Geometry check sheet. Reference: the model listing, model coordinates, mm. Face numbers are marked on the shaded views. A direction names the side the tool comes from. Round coordinates to 2 decimals unless told otherwise and drop trailing zeros. Write each loop counter-clockwise with the first axis right and the second up, starting at its lowest first coordinate (ties: lowest second). Pieces come first, ordered by that corner, then holes. Notation, with made-up numbers: M 42.5,18 L 63.5,18 A26 ccw 63.5,42 Z; hole C -35.5,4 d10. An arc over 180 degrees is marked long. One line per item, written item: value. Start each with the question number.
1. Scan lines: probe 1 along X at (y, z) = (20.5, 17); probe 2 along Z at (x, y) = (8, 2); probe 3 along Y at (x, z) = (33, -2). Record each from-to range of solid material in increasing order. Write a range as [from, to].
2. Depth check by flat-ended pin: P1, Ø12.5, axis at x = 16.5, z = -32, coming from the +Y side; P2, Ø1.1, axis at x = 42.5, z = -40, coming from the -Y side. Enter the tip coordinate at first touch or a pass-through.
3. Access from +Z, -Z, +X, -X, +Y, -Y to the whole of each face (thin tool, end or side, straight path). Record for the marked faces 1 and 2.
4. Section check A-A (x = -21.8). Record the boundary of the cut face in (y, z), and give its area (3 significant figures).
5. Section check C-C (y = 14.5). Count the separate pieces of the cut face and the enclosed holes in it, and give its area (3 significant figures).
6. Section check B-B (z = -6.5). Record the boundary of the cut face in (x, y), and give its area (3 significant figures).
7. Section check D-D (x = 33). Record the boundary of the cut face in (y, z).
8. Release check for a two-part mould opening along X. For the marked faces 3, 4, 5 and 6 record: pulls with the +X half, pulls with the -X half, needs draft (parallel to the pull), parting line crosses it, or undercut.
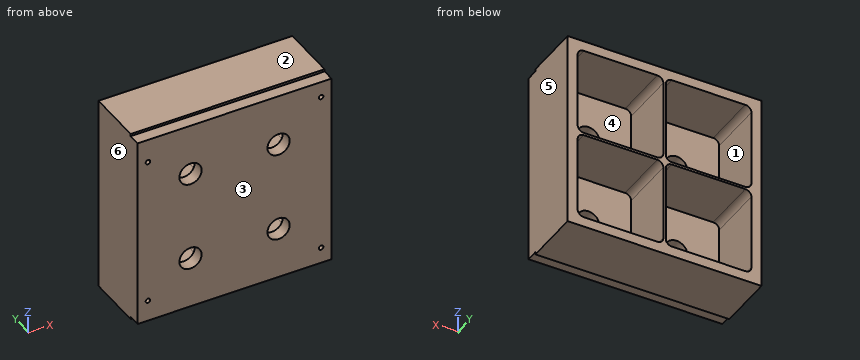
from build123d import *

# Parameters (mm, degrees)
SKETCH1_W           = 96
SKETCH1_H           = 98.4
BOSS_EXTRUDE1_DEPTH = 28
FILLET1_R           = 3
SKETCH2_W           = 96
SKETCH2_H           = 96
BOSS_EXTRUDE2_DEPTH = 6
SKETCH4_R           = 1.1305
CUT_EXTRUDE2_DEPTH  = 4.7
SKETCH6_R           = 5.5
CUT_EXTRUDE3_DEPTH  = 75.22021288


with BuildPart() as part:
    # Sketch1 → Boss-Extrude1 (new body)
    with BuildSketch(Plane(origin=(0, 0, 0), x_dir=(1, 0, 0), z_dir=(0, 1, 0))):
        Rectangle(SKETCH1_W, SKETCH1_H)
        Polygon((-43, -44.2), (-43, -0.6), (-0.6, -0.615), (-0.6, -44.2), align=None, mode=Mode.SUBTRACT)
        Polygon((-43, 44.2), (-0.6, 44.2), (-0.6, 0.615), (-43, 0.6), align=None, mode=Mode.SUBTRACT)
        Polygon((43, -44.2), (43, -0.6), (0.6, -0.615), (0.6, -44.2), align=None, mode=Mode.SUBTRACT)
        Polygon((0.6, 44.2), (43, 44.2), (43, 0.6), (0.6, 0.615), align=None, mode=Mode.SUBTRACT)
    extrude(amount=BOSS_EXTRUDE1_DEPTH)

    # Fillet1
    fillet1_edges = [part.edges().sort_by_distance(p)[0] for p in [
        (-43, 14, 44.2),
        (-0.6, 14, 44.2),
        (-0.6, 14, 0.615),
        (-43, 14, 0.6),
        (-43, 14, -44.2),
        (-43, 14, -0.6),
        (-0.6, 14, -0.615),
        (-0.6, 14, -44.2),
        (43, 14, -0.6),
        (43, 14, -44.2),
        (0.6, 14, -44.2),
        (0.6, 14, -0.615),
        (0.6, 14, 44.2),
        (43, 14, 44.2),
        (43, 14, 0.6),
        (0.6, 14, 0.615),
    ]]
    fillet(fillet1_edges, radius=FILLET1_R)

    # Sketch2 → Boss-Extrude2 (add)
    with BuildSketch(Plane.XZ):
        Rectangle(SKETCH2_W, SKETCH2_H)
    extrude(amount=BOSS_EXTRUDE2_DEPTH)

    # Sketch4 → Cut-Extrude2 (cut)
    with BuildSketch(Plane.XZ.offset(6)):
        with Locations(Location((42.865, -40.005, 0), (0, 0, 270))):
            Circle(SKETCH4_R)
        with Locations(Location((-42.865, -37.465, 0), (0, 0, 270))):
            Circle(SKETCH4_R)
        with Locations(Location((42.865, 40.005, 0), (0, 0, 270))):
            Circle(SKETCH4_R)
        with Locations(Location((-42.865, 36.195, 0), (0, 0, 270))):
            Circle(SKETCH4_R)
    extrude(amount=-CUT_EXTRUDE2_DEPTH, mode=Mode.SUBTRACT)

    # Sketch6 → Cut-Extrude3 (cut, through all)
    with BuildSketch(Plane(origin=(0, 0, 0), x_dir=(1, 0, 0), z_dir=(0, 1, 0))):
        with Locations(Location((-21.8, 22.400530754, 0), (0, 0, 270))):
            Circle(SKETCH6_R)
        with Locations(Location((21.8, 22.400530754, 0), (0, 0, 270))):
            Circle(SKETCH6_R)
        with Locations(Location((21.8, -22.400530754, 0), (0, 0, 270))):
            Circle(SKETCH6_R)
        with Locations(Location((-21.8, -22.400530754, 0), (0, 0, 270))):
            Circle(SKETCH6_R)
    extrude(amount=-CUT_EXTRUDE3_DEPTH, mode=Mode.SUBTRACT)


solid = part.part
Result sheet:
1. probe 1: x = [-48, -43], [-0.6, 0.6], [43, 48]
1. probe 2: z = [-49.2, -44.2], [-0.61, 0.61], [44.2, 49.2]
1. probe 3: y = [-6, 0]
2. P1: stops at y = 0
2. P2: stops at y = -1.3
3. face 1: +Y
3. face 2: +Z, +X, -X, +Y, -Y
4. outline: M -6,-48 L 0,-48 L 0,-49.2 L 28,-49.2 L 28,-44.2 L 0,-44.2 L 0,-27.9 L -6,-27.9 Z; M -6,-16.9 L 0,-16.9 L 0,-0.61 L 28,-0.61 L 28,0.61 L 0,0.61 L 0,16.9 L -6,16.9 Z; M -6,27.9 L 0,27.9 L 0,44.2 L 28,44.2 L 28,49.2 L 0,49.2 L 0,48 L -6,48 Z
4. area: 758 mm2
5. separate pieces: 1
5. enclosed holes: 4
5. area: 2,080 mm2
6. outline: M -48,-6 L 48,-6 L 48,28 L 43,28 L 43,0 L 0.6,0 L 0.6,28 L -0.6,28 L -0.6,0 L -43,0 L -43,28 L -48,28 Z
6. area: 890 mm2
7. outline: M -6,-48 L 0,-48 L 0,-49.2 L 28,-49.2 L 28,-44.2 L 0,-44.2 L 0,-0.6 L 28,-0.6 L 28,0.6 L 0,0.6 L 0,44.2 L 28,44.2 L 28,49.2 L 0,49.2 L 0,48 L -6,48 Z
8. face 3: needs draft
8. face 4: undercut
8. face 5: pulls with the +X half
8. face 6: pulls with the -X half
